Build history of the part. All positions in model axes, mm. Give positions to 0.01 mm unless a question says otherwise; leave off trailing zeros. Loops run counter-clockwise (first coordinate to the right, second up) from the corner with the lowest first, then second, coordinate; pieces in that order, holes last. Notation, with made-up numbers: M 47.25,-33 L 70.25,-33 A26 cw 70.25,-8 Z; hole C 39,88 d9. An arc over 180 degrees is marked long. Answer as a JSON object with one key per item and string values. Group by question number.
1. Drop flat-ended pins along their axis: pin 1 Ø5 at (x, y) = (-31.115, -31.115) entering from -Z; pin 2 Ø9 at (x, y) = (31.115, -31.115) entering from +Z. Give the stop position or say it passes through.
2. Drill centre lines: line 1 along Y through (x, z) = (32, 0.6); line 2 along X through (y, z) = (33.5, 0.15). Where is each one in solid material? Low to high. Write a range as [from, to].
3. Slice it at C-C (y = -22). List the corners of the cut face in (x, z).
4. Slice it at A-A (x = 31). List the corners of the cut face in (y, z), then the cut area to 3 significant figures.
5. Slice it at B-B (z = 0.55). List the corners of the cut face in (x, y) (1 decimal).
6. Mould opens along X. For faces 1 (the face through (-34.22, -34.26, 0.63)), 2 (the face through (38.07, -21.95, 0.63)), 3 (the face through (-1, 1, 1.27)), 4 (the face through (28.847, -29.376, 0.626)) say: released by +X, released by -X, zero draft, split by the parting line, or undercut.
7. Slice it at D-D (x = 18.5). List the corners of the cut face in (y, z).
Autodesk Inventor part; units mm, degrees
ref_plane "YZ Plane" through (0, 0, 0) normal (1, 0, 0) x (0, 1, 0)
ref_plane "XZ Plane" through (0, 0, 0) normal (0, 1, 0) x (-1, 0, 0)
ref_plane "XY Plane" through (0, 0, 0) normal (0, 0, 1) x (1, 0, 0)
sketch "Sketch1" plane through (0, 0, 0) normal (0, 0, 1) x (1, 0, 0)
  circle A0 centre (31.115, 31.115) radius 2.8575
  line L0 (35.0538, 32.8409) -> (41.0029, 11.3509)
  arc A1 (35.0538, 32.8409) -> (32.8409, 35.0538) centre (31.9938, 31.9938) ccw
  line L1 (11.3509, 41.0029) -> (32.8409, 35.0538)
  arc A2 (41.0029, -11.3509) -> (41.0029, 11.3509) centre (0, 0) ccw
  line L2 (41.0029, -11.3509) -> (35.0538, -32.8409)
  line L3 (32.8409, -35.0538) -> (11.3509, -41.0029)
  arc A3 (32.8409, -35.0538) -> (35.0538, -32.8409) centre (31.9938, -31.9938) ccw
  arc A4 (-11.3509, -41.0029) -> (11.3509, -41.0029) centre (0, 0) ccw
  line L4 (-11.3509, -41.0029) -> (-32.8409, -35.0538)
  arc A5 (-35.0538, -32.8409) -> (-32.8409, -35.0538) centre (-31.9938, -31.9938) ccw
  line L5 (-35.0538, -32.8409) -> (-41.0029, -11.3509)
  arc A6 (-41.0029, 11.3509) -> (-41.0029, -11.3509) centre (0, 0) ccw
  line L6 (-41.0029, 11.3509) -> (-35.0538, 32.8409)
  arc A7 (-32.8409, 35.0538) -> (-35.0538, 32.8409) centre (-31.9938, 31.9938) ccw
  line L7 (-32.8409, 35.0538) -> (-11.3509, 41.0029)
  circle A8 centre (-31.115, 31.115) radius 2.8575
  circle A9 centre (-31.115, 31.115) radius 1.5875
  circle A10 centre (31.115, 31.115) radius 1.5875
  circle A11 centre (31.115, -31.115) radius 2.8575
  circle A12 centre (31.115, -31.115) radius 1.5875
  circle A13 centre (-31.115, -31.115) radius 2.8575
  circle A14 centre (-31.115, -31.115) radius 1.5875
  arc A15 (11.3509, 41.0029) -> (-11.3509, 41.0029) centre (0, 0) ccw
  point P0 (0, 0)
extrude "Extrusion1" add sketch "Sketch1" along normal blind 1.27 contours L0 A2 L2 A3 L3 A4 L4 A5 L5 A6 L6 A7 L7 A15 L1 A1
properties part number "Back Plate 1764"
Established:
{
 "1": {"pin 1": "passes through", "pin 2": "stops at z = 1.27"},
 "2": {"line 1": "y = [-35.29, -33.83], [-28.4, 28.4], [33.83, 35.29]", "line 2": "x = [-34.79, -32.69], [-29.54, 29.54], [32.69, 34.79]"},
 "3": {"outline": "M -38.05,0 L 38.05,0 L 38.05,1.27 L -38.05,1.27 Z"},
 "4": {"outline": "M -35.56,0 L -33.97,0 L -33.97,1.27 L -35.56,1.27 Z; M -28.26,0 L 28.26,0 L 28.26,1.27 L -28.26,1.27 Z; M 33.97,0 L 35.56,0 L 35.56,1.27 L 33.97,1.27 Z", "area": "75.8 mm^2"},
 "5": {"outline": "M -41,-11.4 L -35.1,-32.8 A3.2 ccw -32.8,-35.1 L -11.4,-41 A42.5 ccw 11.4,-41 L 32.8,-35.1 A3.2 ccw 35.1,-32.8 L 41,-11.4 A42.5 ccw 41,11.4 L 35.1,32.8 A3.2 ccw 32.8,35.1 L 11.4,41 A42.5 ccw -11.4,41 L -32.8,35.1 A3.2 ccw -35.1,32.8 L -41,11.4 A42.5 ccw Z; hole C -31.1,-31.1 d5.7; hole C -31.1,31.1 d5.7; hole C 31.1,-31.1 d5.7; hole C 31.1,31.1 d5.7"},
 "6": {"face 1": "released by -X", "face 2": "released by +X", "face 3": "zero draft", "face 4": "undercut"},
 "7": {"outline": "M -39.02,0 L 39.02,0 L 39.02,1.27 L -39.02,1.27 Z"}
}
